For this review, take the finished solid that the model builds, in its own axes (mm). Face numbers are marked on the shaded views. A direction names the side the tool comes from. Give positions to 0.01 mm unless a question says otherwise; leave off trailing zeros. Loops run counter-clockwise (first coordinate to the right, second up) from the corner with the lowest first, then second, coordinate; pieces in that order, holes last.
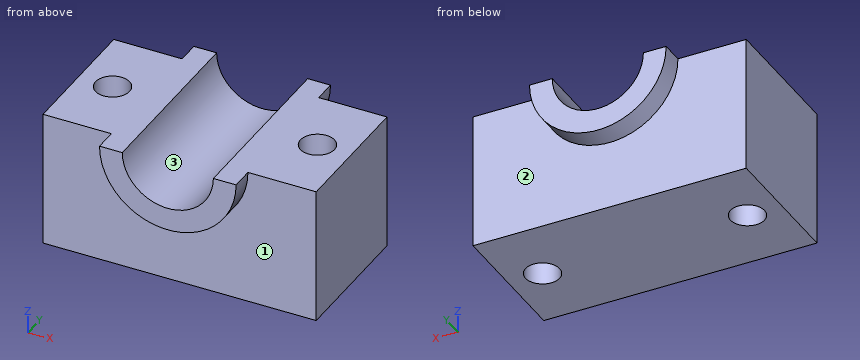
```python
from build123d import *

# Parameters (mm, degrees)
F1_DEPTH      = 38.1
F3_DEPTH      = 12.7
F3_DEPTH_BACK = 88.9
F4_R          = 9.525
F5_R          = 9.525
F6_DEPTH      = 113.03


with BuildPart() as f1:
    # F0 (on Front) → F1 (new body, symmetric)
    with BuildSketch(Plane.XZ):
        with BuildLine():
            Line((-76.2, 38.1), (-76.2, -38.1))
            Line((-76.2, -38.1), (76.2, -38.1))
            Line((76.2, -38.1), (76.2, 38.1))
            Line((76.2, 38.1), (38.1, 38.1))
            ThreePointArc((38.1, 38.1), (0, 0), (-38.1, 38.1))
            Line((-38.1, 38.1), (-76.2, 38.1))
        make_face()
    extrude(amount=F1_DEPTH, both=True)

    # F2 (on face) → F3 (join, two sides)
    with BuildSketch(Plane.XZ.offset(38.1)) as f3_sk:
        with BuildLine():
            Line((-25.4, 38.1), (-38.1, 38.1))
            ThreePointArc((-38.1, 38.1), (0, 0), (38.1, 38.1))
            Line((38.1, 38.1), (25.4, 38.1))
            ThreePointArc((25.4, 38.1), (0, 12.7), (-25.4, 38.1))
        make_face()
    extrude(amount=F3_DEPTH)
    extrude(f3_sk.sketch, amount=-F3_DEPTH_BACK)

    # F4 (on face) + F5 (on face) → F6 (cut)
    with BuildSketch(Plane.XY.offset(38.1)):
        with Locations((-57.15, 0)):
            Circle(F4_R)
    with BuildSketch(Plane.XY.offset(38.1)):
        with Locations((57.15, 0)):
            Circle(F5_R)
    extrude(amount=-F6_DEPTH, mode=Mode.SUBTRACT)


solid = f1.part
```
Item 1: Take a section at D-D on z = 5. Give the boundary of the cut face in (x, y) (3 decimals), and give its area (3 significant figures).
Answer:
outline: (-76.2, -38.1) - (-18.868, -38.1) - (-18.868, -50.8) - (18.868, -50.8) - (18.868, -38.1) - (76.2, -38.1) - (76.2, 38.1) - (18.868, 38.1) - (18.868, 50.8) - (-18.868, 50.8) - (-18.868, 38.1) - (-76.2, 38.1) - close; hole circle Ø19.05 at (-57.15, 0); hole circle Ø19.05 at (57.15, 0)
area: 12,000 mm2
Item 2: For L1, parallel to Y at x = 57, z = -15; L2, parallel to X at y = 4, z = -5; L3, parallel to X at y = -3.5, z = -17, list the stretches that pass through material, from the lowest coordinate up.
Answer:
L1: y = -38.1 to -9.52, 9.52 to 38.1
L2: x = -76.2 to -65.79, -48.51 to 48.51, 65.79 to 76.2
L3: x = -76.2 to -66.01, -48.29 to 48.29, 66.01 to 76.2
Item 3: Take a section at C-C on x = 57.15. Give the boundary of the cut face in (y, z) (3 decimals), and give its area (3 significant figures).
Answer:
outline: (-38.1, -38.1) - (-9.525, -38.1) - (-9.525, 38.1) - (-38.1, 38.1) - close; (9.525, -38.1) - (38.1, -38.1) - (38.1, 38.1) - (9.525, 38.1) - close
area: 4,350 mm2
Item 4: Tool access review of the marked faces 1, 2 and 3: name each direction out of +Z, -Z, +X, -X, +Y, -Y from which nothing blocks a thin tool from reaching the whole face with its end or side.
Answer:
face 1: -Z, -Y
face 2: -Z, +Y
face 3: +Z, +Y, -Y
Item 5: Clearance check with flat-ended pins moving along their axes: pin 1 Ø6 at (x, y) = (7.5, -15.5) entering from +Z; pin 2 Ø8 at (x, z) = (44.5, -13) entering from -Y; pin 3 Ø25 at (x, y) = (-57.15, 0) entering from +Z. State where each tip first meets the part, or that it passes through.
Answer:
pin 1: stops at z = 14.97
pin 2: stops at y = -38.1
pin 3: stops at z = 38.1
Item 6: Take a section at A-A on y = 0. Give the boundary of the cut face in (x, z) (3 decimals), and give its area (3 significant figures).
Answer:
outline: (-76.2, -38.1) - (-66.675, -38.1) - (-66.675, 38.1) - (-76.2, 38.1) - close; (-47.625, -38.1) - (47.625, -38.1) - (47.625, 38.1) - (25.4, 38.1) arc R25.4 cw to (-25.4, 38.1) - (-47.625, 38.1) - close; (66.675, -38.1) - (76.2, -38.1) - (76.2, 38.1) - (66.675, 38.1) - close
area: 7,700 mm2
Item 7: Take a section at B-B on z = 32. State how many separate pieces and enclosed holes the cut face has, and give its area (3 significant figures).
Answer:
separate pieces: 2
enclosed holes: 2
area: 7,940 mm2
